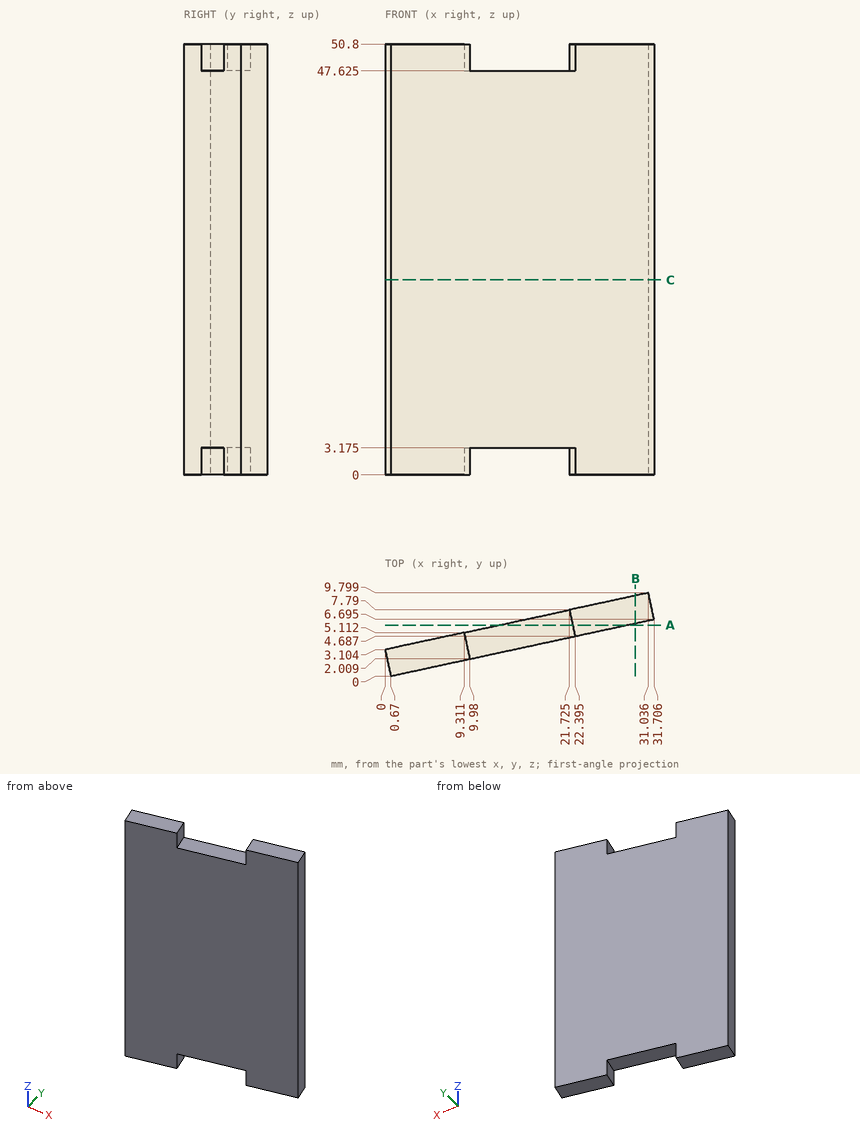
Check sheet for the drawn part. Datum: minimum x, y, z corner. Units: mm. Round coordinates to 2 decimals unless told otherwise and drop trailing zeros. Order: outer loops, then holes, each group sorted by start corner. A loop starts at its lowest first (then second) coordinate and runs counter-clockwise, first axis right, second up. Notation, with made-up numbers: (37.5, 57) -> (52.5, 57) arc R22 cw to (52.5, 83) -> close; hole circle Ø5 at (45, 32.5). An arc over 180 degrees is marked (long way). Use CSV: the item, a comma, the result in double quotes.
(1) Cross-section at C-C (z = 23). Record the boundary of the cut face in (x, y) (1 decimal), and give its area (3 significant figures).
Worked out:
outline,"(0, 3.1) -> (0.7, 0) -> (31.7, 6.7) -> (31, 9.8) -> close"
area,"101 mm²"
(2) Cross-section at B-B (x = 29.5). Record the boundary of the cut face in (y, z), and give its area (3 significant figures).
Worked out:
outline,"(6.22, 0) -> (9.47, 0) -> (9.47, 50.8) -> (6.22, 50.8) -> close"
area,"165 mm²"
(3) Depth check by flat-ended pin: pin 1 (1 mm diameter, centred on x = 13.5, y = 7.5, fed in from +Z); pin 2 (4.5 mm diameter, centred on x = 16, y = 5.5, fed in from +Z) (3 decimals); pin 3 (4 mm diameter, centred on x = 20, y = 3, fed in from -Z) (3 decimals); pin 4 (5 mm diameter, centred on x = 22, z = 6, fed in from +Y). Enter the tip coordinate at first touch or a pass-through.
Worked out:
pin 1,"through"
pin 2,"z = 47.625"
pin 3,"z = 3.175"
pin 4,"y = 8.39"
(4) Cross-section at A-A (y = 6). Record the boundary of the cut face in (x, z) (1 decimal).
Worked out:
outline,"(13.4, 3.2) -> (22.1, 3.2) -> (22.1, 0) -> (28.5, 0) -> (28.5, 50.8) -> (22.1, 50.8) -> (22.1, 47.6) -> (13.4, 47.6) -> close"
(5) Material ranges on line 1 along Z through (x, y) = (18, 6) (1 decimal); line 2 along Y through (x, z) = (25, 3.5); line 3 along Y through (x, z) = (4, 7), recorded low to high. Write a range as from..to.
Worked out:
line 1,"3.2..47.6"
line 2,"5.25..8.5"
line 3,"0.72..3.97"
